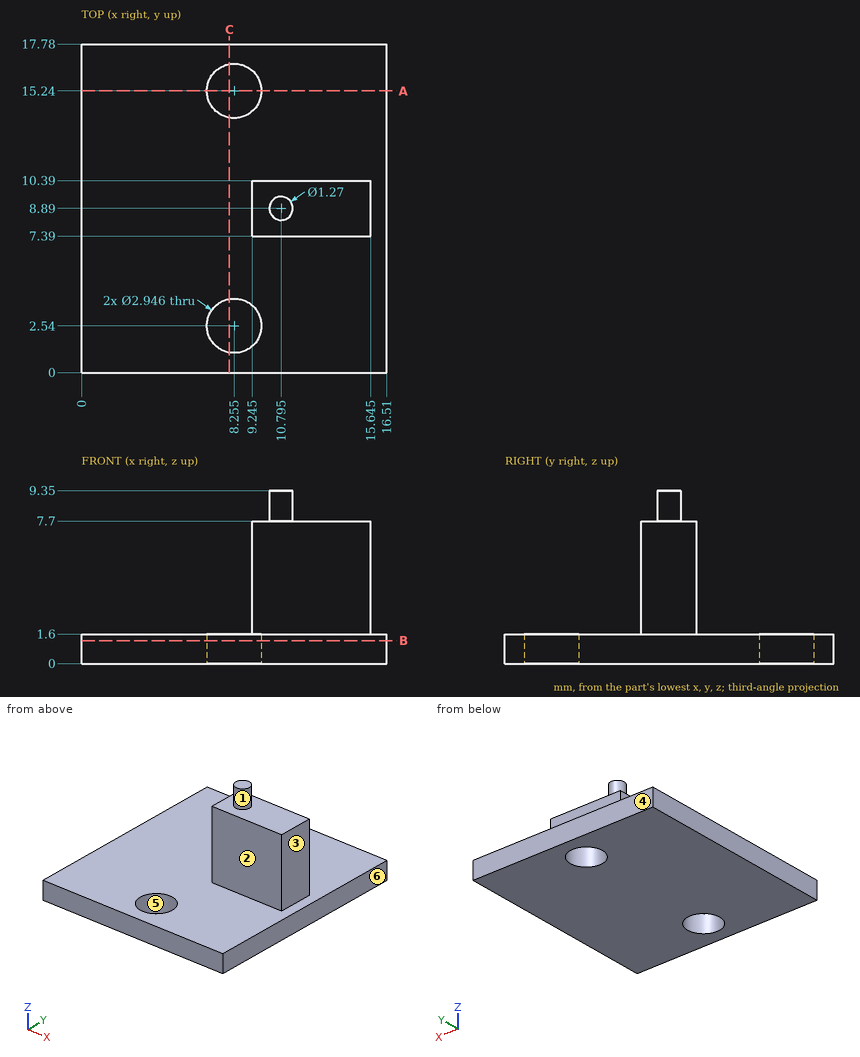
Answer from the drawing. Dimensions are ordinates in mm from the lowest x, y and z of the part. A direction names the side the tool comes from. Coordinates: 2 decimals unless noted, no trailing zeros. Loops run counter-clockwise (first coordinate to the right, second up) from the corner with the lowest first, then second, coordinate; pieces in that order, holes last. Notation, with made-up numbers: (60.25, 75.25) - (117.25, 75.25) arc R3 cw to (117.25, 79.25) - close; hole circle Ø9 at (20, 1). An arc over 180 degrees is marked (long way). Answer in a Markdown table with one row per item.
1. Given pin 1 (3 mm diameter, centred on y = 9, z = 6, fed in from +X) (3 decimals); pin 2 (2 mm diameter, centred on y = 2, z = 3, fed in from -X) (3 decimals); pin 3 (4.5 mm diameter, centred on x = 8.255, y = 15.24, fed in from -Z); pin 4 (3 mm diameter, centred on x = 13.5, z = 6, fed in from +Y), each flat-ended and moving along its own axis, determine where each tip first touches the part or whether it passes through.
Conclusion:
| item | result |
|---|---|
| pin 1 | stops at x = 15.645 |
| pin 2 | passes through |
| pin 3 | stops at z = 0 |
| pin 4 | stops at y = 10.39 |
2. Which of the six approach directions +Z, -Z, +X, -X, +Y, -Y give full straight-line access (tool end or side, diameter ignored) to the marked faces 1, 2 and 3?
Conclusion:
| item | result |
|---|---|
| face 1 | +Z |
| face 2 | +Z, +X, -X, -Y |
| face 3 | +Z, +X, +Y, -Y |
3. Find section B-B, the plane z = 1.25. Write down the section's boundary in (x, y) (1 decimal).
Conclusion:
| item | result |
|---|---|
| outline | (0, 0) - (16.5, 0) - (16.5, 17.8) - (0, 17.8) - close; hole circle Ø2.9 at (8.3, 2.5); hole circle Ø2.9 at (8.3, 15.2) |
4. Straight lines are drawn through the part: line 1 (Y direction, x = 15.5, z = 1.75); line 2 (Z direction, x = 16.25, y = 8.5); line 3 (Z direction, x = 12.5, y = 8.25). For each, find the intervals that lie inside material, in ascending order.
Conclusion:
| item | result |
|---|---|
| line 1 | y = 7.39 to 10.39 |
| line 2 | z = 0 to 1.6 |
| line 3 | z = 0 to 7.7 |
5. Determine the mould class of the marked faces 4, 5 and 6 for opening direction Y: +Y half, -Y half, draft (parallel to the pull), parting line (faces both ways), or undercut.
Conclusion:
| item | result |
|---|---|
| face 4 | +Y half |
| face 5 | undercut |
| face 6 | draft |
6. Find section A-A, the plane y = 15.24. Write down the section's boundary in (x, z).
Conclusion:
| item | result |
|---|---|
| outline | (0, 0) - (6.78, 0) - (6.78, 1.6) - (0, 1.6) - close; (9.73, 0) - (16.51, 0) - (16.51, 1.6) - (9.73, 1.6) - close |
7. Find section C-C, the plane x = 8. Write down the section's boundary in (y, z).
Conclusion:
| item | result |
|---|---|
| outline | (0, 0) - (1.09, 0) - (1.09, 1.6) - (0, 1.6) - close; (3.99, 0) - (13.79, 0) - (13.79, 1.6) - (3.99, 1.6) - close; (16.69, 0) - (17.78, 0) - (17.78, 1.6) - (16.69, 1.6) - close |
